Build history of the part. All positions in model axes, mm. A direction names the side the tool comes from. Give positions to 0.01 mm unless a question says otherwise; leave off trailing zeros. Loops run counter-clockwise (first coordinate to the right, second up) from the corner with the lowest first, then second, coordinate; pieces in that order, holes last. Notation, with made-up numbers: (26, 72.25) - (39, 72.25) arc R28 cw to (39, 91.25) - close; hole circle Ø5 at (23, 3.25). An arc over 180 degrees is marked (long way). Return JSON: item names as keys, results as strings. Group by question number.
1) Slice it at A-A (x = 14.25). List the corners of the cut face in (y, z).
2) Mould opens along X. For faces 1 (the face through (7.301, 187.117, 4.507)), 2 (the face through (10, 193, 6)), 3 (the face through (7.971, 194.314, 2.958)) say: released by +X, released by -X, zero draft, split by the parting line, or undercut.
3) Slice it at C-C (z = -0.5). Count the separate pieces of the cut face and the enclosed holes in it, and give its area (3 significant figures).
4) 3-axis set-ups, long thin cutter, end or side, ignore diameter. For faces 4 (the face through (8, 194, -1)), 5 (the face through (8, 190, 4)), 6 (the face through (0.265, 181, -1)): which of +Z, -Z, +X, -X, +Y, -Y reach the whole face in a straight line?
5) Slice it at D-D (x = 2.5). List the corners of the cut face in (y, z), and give its area (3 significant figures).
6) Drop flat-ended pins along their axis: pin 1 (1.3 mm diameter, centred on x = 14.3, y = 173.68, fed in from -Z); pin 2 (7.5 mm diameter, centred on x = 8.5, y = 178.5, fed in from +Z); pin 3 (3 mm diameter, centred on x = 7.87, y = 189.68, fed in from +Z); pin 4 (1.3 mm diameter, centred on x = 9.5, z = -0.5, fed in from +Y). Give the stop position or say it passes through.
7) Slice it at B-B (y = 183.25). List the corners of the cut face in (x, z), and give its area (3 significant figures).
8) Drill centre lines: probe 1 along Y at (x, z) = (14.75, -1); probe 2 along Z at (x, y) = (11, 177.5); probe 3 along Y at (x, z) = (7, 4.5). Where is each one in solid material? Low to high. Write a range as from..to.
```python
from build123d import *

# Parameters (mm, degrees)
ESQUISSE1_W             = 15.163065961
ESQUISSE1_H             = 24.718099935
ESQUISSE1_R             = 1.620437073
ESQUISSE1_R_2           = 1.629155484
ESQUISSE1_R_3           = 0.551783112
BOSS_EXTRU_1_DEPTH      = 1.6
ESQUISSE2_R             = 4.635270965
BOSS_EXTRU_2_DEPTH      = 6
ESQUISSE3_R             = 2.625763286
ENL_V_MAT_EXTRU_1_DEPTH = 2
CHANFREIN1_SIZE         = 1


with BuildPart() as part:
    # Esquisse1 → Boss.-Extru.1 (new body)
    with BuildSketch(Plane.XY):
        with Locations((7.846483978, 181.640524959)):
            Rectangle(ESQUISSE1_W, ESQUISSE1_H)
        with Locations((2.740050159, 183.860713577)):
            Circle(ESQUISSE1_R, mode=Mode.SUBTRACT)
        with Locations((12.98580948, 183.819598973)):
            Circle(ESQUISSE1_R_2, mode=Mode.SUBTRACT)
        with Locations((1.503458801, 178.757435176)):
            Circle(ESQUISSE1_R_3, mode=Mode.SUBTRACT)
        with Locations((1.490795777, 176.217466742)):
            Circle(ESQUISSE1_R_3, mode=Mode.SUBTRACT)
        with Locations((1.478132752, 173.677498307)):
            Circle(ESQUISSE1_R_3, mode=Mode.SUBTRACT)
        with Locations((1.465469727, 171.137529873)):
            Circle(ESQUISSE1_R_3, mode=Mode.SUBTRACT)
        with Locations(Location((14.313761483, 171.137529873, 0), (0, 0, 180))):
            Circle(ESQUISSE1_R_3, mode=Mode.SUBTRACT)
        with Locations(Location((14.301098459, 173.677498307, 0), (0, 0, 180))):
            Circle(ESQUISSE1_R_3, mode=Mode.SUBTRACT)
        with Locations(Location((14.288435434, 176.217466742, 0), (0, 0, 180))):
            Circle(ESQUISSE1_R_3, mode=Mode.SUBTRACT)
        with Locations(Location((14.275772409, 178.757435176, 0), (0, 0, 180))):
            Circle(ESQUISSE1_R_3, mode=Mode.SUBTRACT)
    extrude(amount=-BOSS_EXTRU_1_DEPTH)

    # Esquisse2 → Boss.-Extru.2 (add)
    with BuildSketch(Plane.XY):
        with Locations(Location((7.870027941, 189.680070203, 0), (0, 0, 111.270599652))):
            Circle(ESQUISSE2_R)
    extrude(amount=BOSS_EXTRU_2_DEPTH)

    # Esquisse3 → Enlèv. mat.-Extru.1 (cut)
    with BuildSketch(Plane.XY.offset(6)):
        with Locations((7.870027941, 189.680070203)):
            Circle(ESQUISSE3_R)
    extrude(amount=-ENL_V_MAT_EXTRU_1_DEPTH, mode=Mode.SUBTRACT)

    # Chanfrein1
    chanfrein1_edges = [part.edges().sort_by_distance(p)[0] for p in [
        (5.244264654, 189.680070203, 6),
    ]]
    chamfer(chanfrein1_edges, length=CHANFREIN1_SIZE)


solid = part.part
```
Results:
{
 "1": {"outline": "(169.28, -1.6) - (170.59, -1.6) - (170.59, 0) - (169.28, 0) - close; (171.69, -1.6) - (173.13, -1.6) - (173.13, 0) - (171.69, 0) - close; (174.23, -1.6) - (175.67, -1.6) - (175.67, 0) - (174.23, 0) - close; (176.77, -1.6) - (178.21, -1.6) - (178.21, 0) - (176.77, 0) - close; (179.31, -1.6) - (182.79, -1.6) - (182.79, 0) - (179.31, 0) - close; (184.85, -1.6) - (194, -1.6) - (194, 0) - (184.85, 0) - close"},
 "2": {"face 1": "undercut", "face 2": "zero draft", "face 3": "split by the parting line"},
 "3": {"separate pieces": "1", "enclosed holes": "10", "area": "351 mm2"},
 "4": {"face 4": "-Z, +X, -X, +Y", "face 5": "+Z", "face 6": "+Z, -Z, -X, +Y, -Y"},
 "5": {"outline": "(169.28, -1.6) - (182.26, -1.6) - (182.26, 0) - (169.28, 0) - close; (185.46, -1.6) - (194, -1.6) - (194, 0) - (185.46, 0) - close", "area": "34.4 mm2"},
 "6": {"pin 1": "z = -1.6", "pin 2": "z = 0", "pin 3": "z = 4", "pin 4": "y = 194.15"},
 "7": {"outline": "(0.26, -1.6) - (1.24, -1.6) - (1.24, 0) - (0.26, 0) - close; (4.24, -1.6) - (11.46, -1.6) - (11.46, 0) - (4.24, 0) - close; (14.51, -1.6) - (15.43, -1.6) - (15.43, 0) - (14.51, 0) - close", "area": "14.6 mm2"},
 "8": {"probe 1": "169.28..170.8, 171.48..173.36, 174..175.92, 176.52..178.48, 179.04..194", "probe 2": "-1.6..0", "probe 3": "185.13..187.2, 192.16..194.23"}
}
